Input: part model. Units: mm. Frame: model coordinates. A direction names the side the tool comes from. Give positions to 0.01 mm unless a question says otherwise; leave off trailing zeros. Write each loop counter-clockwise with the first axis right and the second up, starting at its lowest first coordinate (ties: lowest second). Pieces come first, ordered by that corner, then holes. Notation, with made-up numbers: (85, 5.5) -> (132, 5.5) arc R25 ccw to (132, 18.5) -> close; hole circle Ø2 at (32.5, 54). An arc over 180 degrees is marked (long way). Answer as a JSON object with one key per item and string values. Group by question number.
from build123d import *

# Parameters (mm, degrees)
SKETCH_1_R          = 5
SKETCH_1_R_2        = 2.5
EXTRUDE_1_DEPTH     = 7
SKETCH_2_R          = 5
SKETCH_2_R_2        = 4
EXTRUDE_2_DEPTH     = 7
FILLET_1_R          = 0.3
SKETCH_3_R          = 1
CUT_EXTRUDE_1_DEPTH = 7


with BuildPart() as part:
    # 草图1 → 凸台-拉伸1 (new body)
    with BuildSketch(Plane(origin=(0, 0, 0), x_dir=(1, 0, 0), z_dir=(0, 1, 0))):
        with Locations(Location((0, 0, 0), (0, 0, 270))):
            Circle(SKETCH_1_R)
        with Locations(Location((0, 0, 0), (0, 0, 270))):
            Circle(SKETCH_1_R_2, mode=Mode.SUBTRACT)
    extrude(amount=EXTRUDE_1_DEPTH)

    # 草图2 → 凸台-拉伸2 (add)
    with BuildSketch(Plane(origin=(0, 7, 0), x_dir=(1, 0, 0), z_dir=(0, 1, 0))):
        with Locations(Location((0, 0, 0), (0, 0, 270))):
            Circle(SKETCH_2_R)
        with Locations(Location((0, 0, 0), (0, 0, 270))):
            Circle(SKETCH_2_R_2, mode=Mode.SUBTRACT)
    extrude(amount=EXTRUDE_2_DEPTH)

    # 圆角1
    fillet_1_edges = [part.edges().sort_by_distance(p)[0] for p in [
        (0, 14, -5),
        (0, 0, -5),
    ]]
    fillet(fillet_1_edges, radius=FILLET_1_R)

    # 草图3 → 切除-拉伸1 (cut)
    with BuildSketch(Plane.XY):
        with Locations(Location((0, 11, 0), (0, 0, 90))):
            Circle(SKETCH_3_R)
        with Locations(Location((0, 3, 0), (0, 0, 90))):
            Circle(SKETCH_3_R)
    extrude(amount=-CUT_EXTRUDE_1_DEPTH, mode=Mode.SUBTRACT)


solid = part.part
1. Contact query for a flat-ended pin moving along its axis: pin 1 Ø2 at (x, y) = (-2.5, 3) entering from +Z. Output: stop coordinate, or through.
2. Section B-B (z = 0). Return the cut outline in (x, y).
3. Mould query, pull axis Y, two halves, no side actions, for faces 1 (the face through (-1, 3, -4)), 2 (the face through (4, 14, 2)), 3 (the face through (0.6, 10.2, -4.4)), 4 (the face through (-2, 0, 2)). Classes: pulls with the +Y half, pulls with the -Y half, needs draft (parallel to the pull), parting line crosses it, or undercut.
4. Line query: line 1 (X direction, y = 4.25, z = 0); line 2 (X direction, y = 11.75, z = 0); line 3 (Y direction, x = 3.5, z = 0.5). Output: solid intervals per line, ascending.
5. Section D-D (y = 3). Return the cut outline in (x, z), plus the area to 3 significant figures.
6. Reachability of faces 5 (the face through (0.751, 3.451, 2.385)), 6 (the face through (-1.532, 10.451, 3.695)) from +Z, -Z, +X, -X, +Y, -Y: full face, straight path, thin tool, end or side. Return the list, or none.
7. Section C-C (y = 1.25). Return the cut outline in (x, z), plus the area to 3 significant figures.
8. Section A-A (x = 0). Return the cut outline in (y, z), plus the area to 3 significant figures.
Working result:
{
 "1": {"pin 1": "stops at z = 4.77"},
 "2": {"outline": "(-5, 0.3) arc R0.3 ccw to (-4.7, 0) -> (-2.5, 0) -> (-2.5, 7) -> (-4, 7) -> (-4, 14) -> (-4.7, 14) arc R0.3 ccw to (-5, 13.7) -> close; (2.5, 0) -> (4.7, 0) arc R0.3 ccw to (5, 0.3) -> (5, 13.7) arc R0.3 ccw to (4.7, 14) -> (4, 14) -> (4, 7) -> (2.5, 7) -> close"},
 "3": {"face 1": "undercut", "face 2": "pulls with the +Y half", "face 3": "undercut", "face 4": "pulls with the -Y half"},
 "4": {"line 1": "x = -5 to -2.5, 2.5 to 5", "line 2": "x = -5 to -4, 4 to 5", "line 3": "y = 0 to 7"},
 "5": {"outline": "(-1, -4.9) -> (-1, -2.29) arc R2.5 cw (long way) to (1, -2.29) -> (1, -4.9) arc R5 ccw (long way) to start", "area": "53.8 mm^2"},
 "6": {"face 5": "+Y, -Y", "face 6": "+Y"},
 "7": {"outline": "circle Ø10 at (0, 0); hole circle Ø5 at (0, 0)", "area": "58.9 mm^2"},
 "8": {"outline": "(0, -4.7) arc R0.3 ccw to (0.3, -5) -> (2, -5) -> (2, -2.5) -> (0, -2.5) -> close; (0, 2.5) -> (7, 2.5) -> (7, 4) -> (14, 4) -> (14, 4.7) arc R0.3 ccw to (13.7, 5) -> (0.3, 5) arc R0.3 ccw to (0, 4.7) -> close; (4, -5) -> (10, -5) -> (10, -4) -> (7, -4) -> (7, -2.5) -> (4, -2.5) -> close; (12, -5) -> (13.7, -5) arc R0.3 ccw to (14, -4.7) -> (14, -4) -> (12, -4) -> close", "area": "41.9 mm^2"}
}
